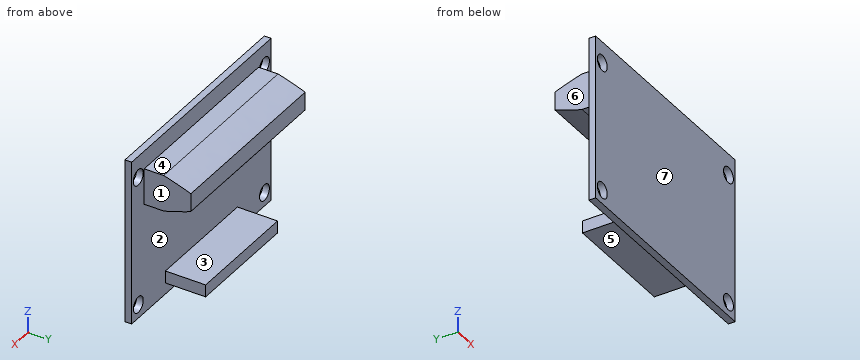
```python
from build123d import *

# Parameters (mm, degrees)
SKETCH1_W           = 49.4
SKETCH1_H           = 36.5
SKETCH1_R           = 1.75
BOSS_EXTRUDE1_DEPTH = 1.5
SKETCH1_3_W         = 40.5
SKETCH1_3_H         = 8
BOSS_EXTRUDE2_DEPTH = 11.8
FILLET1_SIZE        = 6
FILLET1_SIZE_2      = 2
FILLET2_SIZE        = 6
FILLET2_SIZE_2      = 2
SKETCH1_4_W         = 25.5
SKETCH1_4_H         = 2.7
BOSS_EXTRUDE3_DEPTH = 10.4


with BuildPart() as part:
    # Sketch1 → Boss-Extrude1 (new body)
    with BuildSketch(Plane(origin=(0, 0, 0), x_dir=(1, 0, 0), z_dir=(0, 1, 0))):
        with Locations((-101.179682497, -14.992188262)):
            Rectangle(SKETCH1_W, SKETCH1_H)
        with Locations(Location((-123.529682497, 0.207811738, 0), (0, 0, 270))):
            Circle(SKETCH1_R, mode=Mode.SUBTRACT)
        with Locations(Location((-78.829682497, 0.207811738, 0), (0, 0, 270))):
            Circle(SKETCH1_R, mode=Mode.SUBTRACT)
        with Locations(Location((-123.529682497, -28.492188262, 0), (0, 0, 270))):
            Circle(SKETCH1_R, mode=Mode.SUBTRACT)
        with Locations(Location((-78.829682497, -28.492188262, 0), (0, 0, 270))):
            Circle(SKETCH1_R, mode=Mode.SUBTRACT)
    extrude(amount=BOSS_EXTRUDE1_DEPTH)

    # Sketch1<3> → Boss-Extrude2 (add)
    with BuildSketch(Plane(origin=(0, 0, 0), x_dir=(1, 0, 0), z_dir=(0, 1, 0))):
        with Locations((-101.179682497, -25.242188262)):
            Rectangle(SKETCH1_3_W, SKETCH1_3_H)
    extrude(amount=BOSS_EXTRUDE2_DEPTH)

    # Fillet1
    # a fillet whose section is not a circle: 6, 2 mm, written as the material it takes off along each edge
    with BuildSketch(Plane(origin=(-136.429682497, 11.8, 21.242188262), x_dir=(0, -1, 0), z_dir=(1, 0, 0))) as fillet1_piece_1:
        with BuildLine():
            Bezier((FILLET1_SIZE, 0), (0, 0), (0, -FILLET1_SIZE_2), weights=[1, 0.052631579, 1])
            Line((0, -FILLET1_SIZE_2), (0, 0))
            Line((0, 0), (FILLET1_SIZE, 0))
        make_face()
    extrude(amount=70.5, mode=Mode.SUBTRACT)

    # Fillet2
    # a fillet whose section is not a circle: 6, 2 mm, written as the material it takes off along each edge
    with BuildSketch(Plane(origin=(-65.929682497, 11.8, 29.242188262), x_dir=(0, -1, 0), z_dir=(-1, 0, 0))) as fillet2_piece_1:
        with BuildLine():
            Bezier((FILLET2_SIZE, 0), (0, 0), (0, -FILLET2_SIZE_2), weights=[1, 0.052631579, 1])
            Line((0, -FILLET2_SIZE_2), (0, 0))
            Line((0, 0), (FILLET2_SIZE, 0))
        make_face()
    extrude(amount=70.5, mode=Mode.SUBTRACT)

    # Sketch1<4> → Boss-Extrude3 (add)
    with BuildSketch(Plane(origin=(0, 0, 0), x_dir=(1, 0, 0), z_dir=(0, 1, 0))):
        with Locations((-101.179682497, -0.592188262)):
            Rectangle(SKETCH1_4_W, SKETCH1_4_H)
    extrude(amount=BOSS_EXTRUDE3_DEPTH)


solid = part.part
```
Geometry: final body of the model. Coordinates: model frame, mm. Face numbers are marked on the shaded views. A direction names the side the tool comes from. Give positions to 0.01 mm unless a question says otherwise; leave off trailing zeros. Order: outer loops, then holes, each group sorted by start corner. A loop starts at its lowest first (then second) coordinate and runs counter-clockwise, first axis right, second up. Notation, with made-up numbers: (25, -20) -> (39, -20) arc R21 ccw to (39, 4) -> close; hole circle Ø4 at (37.25, -11.5). An arc over 180 degrees is marked (long way). Write each question's results on one line, items separated by ' | '. Start each with the question number.
1) Set-up query: the marked faces 5, 6 and 7. Return all of +Z, -Z, +X, -X, +Y, -Y with unobstructed straight access to the full face (end or side cutting, diameter ignored); none if empty.
2) Draft query along Z for the marked faces 1, 2, 3 and 4. Return one class per face: pulls with the +Z half, pulls with the -Z half, needs draft (parallel to the pull), parting line crosses it, or undercut.
3) First-contact query: pin 1 (0.8 mm diameter, centred on y = 4, z = 1, fed in from -X); pin 2 (2 mm diameter, centred on x = -92.5, y = 4, fed in from -Z); pin 3 (5 mm diameter, centred on x = -113, z = 15.5, fed in from +Y); pin 4 (1 mm diameter, centred on y = 6.5, z = 2.5, fed in from -X). Flat tips, straight axial feed; report the tip coordinate or a pass-through.
4) Section C-C (z = 0). Return loops of the section in (x, y), then the cut area to 3 significant figures.
5) Section A-A (x = -80). Return loops of the section in (y, z).
6) Section D-D (z = 6). Return loops of the section in (x, y), then the cut area to 3 significant figures.
7) Section B-B (y = 2.25). Return loops of the section in (x, z), then the cut area to 3 significant figures.
8) Line query: line 1 (Z direction, x = -100, y = 4); line 2 (Z direction, x = -110.5, y = 6); line 3 (Y direction, x = -118, z = 18). Output: solid intervals per line, ascending. Write a range as from..to.
Calculated:
1) face 5: -Z, +X, -X, +Y | face 6: +Z, -Z, -X, +Y | face 7: +Z, -Z, +X, -X, -Y
2) face 1: needs draft | face 2: undercut | face 3: undercut | face 4: pulls with the +Z half
3) pin 1: x = -113.93 | pin 2: z = -0.76 | pin 3: y = 1.5 | pin 4: through
4) outline: (-125.88, 0) -> (-125.27, 0) -> (-125.27, 1.5) -> (-125.88, 1.5) -> close; (-121.79, 0) -> (-80.57, 0) -> (-80.57, 1.5) -> (-88.43, 1.5) -> (-88.43, 10.4) -> (-113.93, 10.4) -> (-113.93, 1.5) -> (-121.79, 1.5) -> close; (-77.09, 0) -> (-76.48, 0) -> (-76.48, 1.5) -> (-77.09, 1.5) -> close | area: 291 mm2
5) outline: (0, -3.26) -> (1.5, -3.26) -> (1.5, -1.51) -> (0, -1.51) -> close; (0, 1.09) -> (1.5, 1.09) -> (1.5, 27.19) -> (0, 27.19) -> close; (0, 29.79) -> (1.5, 29.79) -> (1.5, 33.24) -> (0, 33.24) -> close
6) outline: (-125.88, 0) -> (-76.48, 0) -> (-76.48, 1.5) -> (-125.88, 1.5) -> close | area: 74.1 mm2
7) outline: (-121.43, 21.24) -> (-80.93, 21.24) -> (-80.93, 29.24) -> (-121.43, 29.24) -> close; (-113.93, -0.76) -> (-88.43, -0.76) -> (-88.43, 1.94) -> (-113.93, 1.94) -> close | area: 393 mm2
8) line 1: -0.76..1.94, 21.24..29.24 | line 2: -0.76..1.94, 21.28..29.2 | line 3: 0..1.5
